Model file for the job. Use its own axes, mm. Face numbers are marked on the shaded views. Round coordinates to 2 decimals unless told otherwise and drop trailing zeros. Loops run counter-clockwise (first coordinate to the right, second up) from the corner with the lowest first, then second, coordinate; pieces in that order, holes last. Notation, with made-up numbers: M -24.5,61 L 13.5,61 A7 cw 13.5,74 Z; hole C 67,16.25 d11. An arc over 180 degrees is marked long. Answer in a Markdown table with one row per item.
Autodesk Inventor part; units mm, degrees
ref_plane "YZ Plane" through (0, 0, 0) normal (1, 0, 0) x (0, 1, 0)
ref_plane "XZ Plane" through (0, 0, 0) normal (0, 1, 0) x (-1, 0, 0)
ref_plane "XY Plane" through (0, 0, 0) normal (0, 0, 1) x (1, 0, 0)
sketch "Sketch1" plane through (0, 0, 0) normal (0, 0, 1) x (1, 0, 0)
  line L0 (0, 0) -> (12.7, 0)
  line L1 (12.7, 0) -> (12.7, 25.4)
  line L2 (12.7, 25.4) -> (0, 25.4)
  line L3 (0, 25.4) -> (0, 0)
  line L4 (6.35, 0) -> (6.35, 6.35)
  circle A0 centre (6.35, 6.35) radius 2.54
  line L5 (6.35, 6.35) -> (6.35, 19.05)
  circle A1 centre (6.35, 19.05) radius 2.54
  dimension "d0" = 12.7
  dimension "d1" = 25.4
  dimension "d2" = 6.35
  dimension "d3" = 5.08
  dimension "d4" = 12.7
  dimension "d5" = 5.08
extrude "Extrusion1" add sketch "Sketch1" along normal blind 1.5875
fillet "Fillet1" radius 3.175 4 edges at (12.7, 25.4, 0.7937) (0, 25.4, 0.7937) (12.7, 0, 0.7937) (0, 0, 0.7937)
properties part number "polySpacer2"
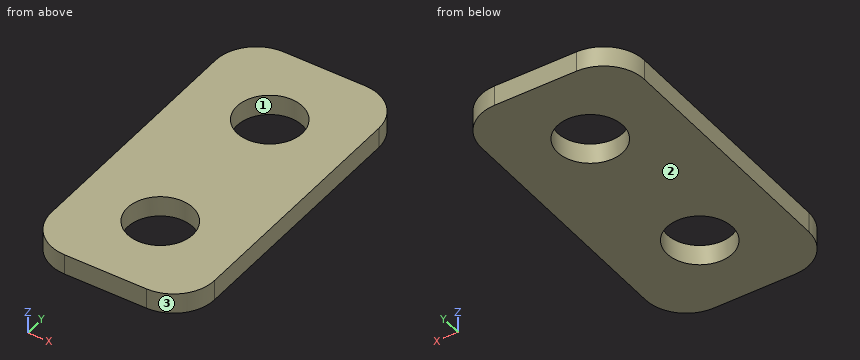
1. Mould opens along X. For the marked faces 1, 2 and 3 say: +X half, -X half, draft (parallel to the pull), parting line (faces both ways), or undercut.
Verdict:
| item | result |
|---|---|
| face 1 | undercut |
| face 2 | draft |
| face 3 | +X half |
2. Saw through at B-B (y = 19.05). Write the cut outline in (x, z), and give its area (3 significant figures).
Verdict:
| item | result |
|---|---|
| outline | M 0,0 L 3.81,0 L 3.81,1.59 L 0,1.59 Z; M 8.89,0 L 12.7,0 L 12.7,1.59 L 8.89,1.59 Z |
| area | 12.1 mm² |
3. Wall check: probe 1 along Y at (x, z) = (6.35, 0.9); probe 2 along Y at (x, z) = (8, 1.05); probe 3 along X at (y, z) = (20.5, 0.5). Give the ranges that are in metal, low to high.
Verdict:
| item | result |
|---|---|
| probe 1 | y = 0 to 3.81, 8.89 to 16.51, 21.59 to 25.4 |
| probe 2 | y = 0 to 4.42, 8.28 to 17.12, 20.98 to 25.4 |
| probe 3 | x = 0 to 4.26, 8.44 to 12.7 |
4. Saw through at C-C (y = 7.75). Write the cut outline in (x, z).
Verdict:
| item | result |
|---|---|
| outline | M 0,0 L 4.23,0 L 4.23,1.59 L 0,1.59 Z; M 8.47,0 L 12.7,0 L 12.7,1.59 L 8.47,1.59 Z |
5. Saw through at D-D (x = 1.5). Write the cut outline in (y, z).
Verdict:
| item | result |
|---|---|
| outline | M 0.48,0 L 24.92,0 L 24.92,1.59 L 0.48,1.59 Z |
6. Saw through at A-A (x = 6.35). Write the cut outline in (y, z), and give its area (3 significant figures).
Verdict:
| item | result |
|---|---|
| outline | M 0,0 L 3.81,0 L 3.81,1.59 L 0,1.59 Z; M 8.89,0 L 16.51,0 L 16.51,1.59 L 8.89,1.59 Z; M 21.59,0 L 25.4,0 L 25.4,1.59 L 21.59,1.59 Z |
| area | 24.2 mm² |
